Autodesk Inventor part; units mm, degrees
ref_plane "YZ Plane" through (0, 0, 0) normal (1, 0, 0) x (0, 1, 0)
ref_plane "XZ Plane" through (0, 0, 0) normal (0, 1, 0) x (-1, 0, 0)
ref_plane "XY Plane" through (0, 0, 0) normal (0, 0, 1) x (1, 0, 0)
sketch "Sketch1" plane through (0, 0, 0) normal (0, 0, 1) x (1, 0, 0)
  arc A0 (0, 10) -> (100, 10) centre (50, 130) ccw
  line L0 (0, 55) -> (13, 55)
  line L1 (13, 55) -> (13, 25)
  line L2 (13, 25) -> (0, 25)
  line L3 (13, 47.5) -> (39, 47.5)
  line L4 (39, 47.5) -> (39, 46)
  line L5 (39, 46) -> (13, 46)
  line L6 (13, 46) -> (13, 47.5)
  line L7 (13, 34) -> (39, 34)
  line L8 (39, 34) -> (39, 32.5)
  line L9 (39, 32.5) -> (13, 32.5)
  line L10 (13, 46) -> (14, 46)
  line L11 (14, 46) -> (14, 44)
  line L12 (14, 44) -> (13, 44)
  line L13 (13, 44) -> (13, 46)
  line L14 (13, 34) -> (14, 34)
  line L15 (14, 34) -> (14, 36)
  line L16 (14, 36) -> (13, 36)
  line L17 (13, 36) -> (13, 34)
  line L18 (30, 150) -> (32, 142)
  arc A1 (32, 142) -> (50, 141) centre (50, 303.5) ccw
  line L19 (100, 55) -> (87, 55)
  line L20 (87, 55) -> (87, 25)
  line L21 (87, 25) -> (100, 25)
  line L22 (87, 47.5) -> (61, 47.5)
  line L23 (61, 47.5) -> (61, 46)
  line L24 (61, 46) -> (87, 46)
  line L25 (87, 46) -> (87, 47.5)
  line L26 (61, 34) -> (61, 32.5)
  line L27 (87, 34) -> (61, 34)
  line L28 (61, 32.5) -> (87, 32.5)
  line L29 (87, 46) -> (86, 46)
  line L30 (86, 46) -> (86, 44)
  line L31 (86, 44) -> (87, 44)
  line L32 (87, 44) -> (87, 46)
  line L33 (87, 34) -> (86, 34)
  line L34 (86, 34) -> (86, 36)
  line L35 (86, 36) -> (87, 36)
  line L36 (87, 36) -> (87, 34)
  line L37 (70, 150) -> (68, 142)
  arc A2 (50, 141) -> (68, 142) centre (50, 303.5) ccw
  arc A3 (100, 55) -> (80, 150) centre (-148.869, 52.2118) ccw
  line L38 (70, 150) -> (80, 150)
  line L39 (20, 150) -> (30, 150)
  line L40 (100, 25) -> (100, 10)
  line L41 (0, 10) -> (0, 25)
  circle A4 centre (25.0045, 134) radius 1.5 construction
  circle A5 centre (74.7045, 134) radius 1.5 construction
  line L42 (16.9872, 134) -> (99.6032, 134) construction
  line L43 (12.0158, 134) -> (23.5045, 134)
  line L44 (74.7045, 134) -> (86.1932, 134)
  circle A6 centre (25.0045, 134) radius 2
  circle A7 centre (74.7045, 134) radius 2
  circle A8 centre (14.98, 88.58) radius 1.5 construction
  circle A9 centre (86.52, 88.58) radius 1.5 construction
  line L45 (16.652, 88.58) -> (99.2681, 88.58) construction
  line L46 (2.6559, 88.58) -> (13.48, 88.58)
  line L47 (86.52, 88.58) -> (97.3441, 88.58)
  circle A10 centre (14.98, 88.58) radius 2
  circle A11 centre (86.52, 88.58) radius 2
  line L48 (13, 50.0336) -> (87, 50.0336) construction
  line L49 (50, 50.0336) -> (50, 74.1687) construction
  arc A12 (20, 150) -> (0, 55) centre (248.869, 52.2118) ccw
  line L50 (0, 27.09) -> (23.905, 27.09)
  circle A13 centre (25.405, 27.09) radius 1.5 construction
  circle A14 centre (25.405, 27.09) radius 2
  circle A15 centre (76.095, 27.09) radius 1.5 construction
  circle A16 centre (76.095, 27.09) radius 2
  line L51 (30.9298, 27.09) -> (113.5459, 27.09) construction
  line L52 (76.095, 27.09) -> (100, 27.09)
  point P0 (0, 0)
  point P1 (75, 150)
  point P2 (50.8983, 94.4188)
  point P3 (62.5692, 16.9025)
  dimension "d68" = 3
  dimension "d74" = 3
  dimension "d80" = 3
  dimension "d10" = 10
  dimension "d12" = 30
  dimension "d13" = 13
  dimension "d14" = 15
  dimension "d15" = 26
  dimension "d16" = 1.5
  dimension "d19" = 26
  dimension "d20" = 1.5
  dimension "d23" = 7.5
  dimension "d24" = 12
  dimension "d25" = 1
  dimension "d26" = 2
  dimension "d27" = 1
  dimension "d28" = 2
  dimension "d35" = 10
  dimension "d69" = 3
  dimension "d70" = 46.7
  dimension "d71" = 16
  dimension "d72" = 4
  dimension "d73" = 4
  dimension "d75" = 3
  dimension "d76" = 68.54
  dimension "d77" = 4
  dimension "d78" = 4
  dimension "d79" = 45.42
  dimension "d81" = 3
  dimension "d83" = 4
  dimension "d84" = 4
  dimension "d86" = 61.49
  dimension "d107" = 46.69
extrude "Extrusion1" add sketch "Sketch1" along normal blind 10 contours L1 L7 L8 L9 | L28 L26 L27 L20 | L1 L16 L15 L7 | L27 L34 L35 L20 | L1 L5 L11 L12 | L31 L30 L24 L20 | L1 L3 L4 L5 | L24 L23 L22 L20
extrude "Extrusion3" add sketch "Sketch1" along normal blind 3 contours L41 L2 L1 L9 L8 L7 L15 L16 L12 L11 L5 L4 L3 L0 A12 L39 L18 A1 A2 L37 L38 A3 L19 L20 L22 L23 L24 L30 L31 L35 L34 L27 L26 L28 L21 L40 A0
sketch "Sketch2" plane through (0, 0, 3) normal (0, 0, 1) x (1, 0, 0)
  line L0 (39, 34) -> (14, 34)
  line L1 (17.3, 34) -> (16.3, 34)
  line L2 (16.3, 34) -> (16.3, 36)
  line L3 (16.3, 36) -> (17.3, 36)
  line L4 (17.3, 36) -> (17.3, 34)
  line L5 (14, 34) -> (14, 36)
  line L6 (61, 46) -> (86, 46)
  line L7 (83.7, 46) -> (82.7, 46)
  line L8 (82.7, 46) -> (82.7, 44)
  line L9 (82.7, 44) -> (83.7, 44)
  line L10 (83.7, 44) -> (83.7, 46)
  line L11 (86, 46) -> (86, 44)
  point P0 (0, 0)
  point P1 (14, 35)
  dimension "d89" = 1
  dimension "d90" = 2
  dimension "d91" = 2.3
  dimension "d92" = 1
  dimension "d93" = 2
  dimension "d94" = 2.3
extrude "Extrusion4" add sketch "Sketch2" along normal blind 1.5
extrude "Extrusion5" add sketch "Sketch1" along normal blind 24 contours A16 | A11 | A7 | A6 | A10 | A14
sketch "Sketch4" plane through (74.7045, 134, 24) normal (0, 0, 1) x (1, 0, 0)
  circle A0 centre (-49.7, 0) radius 2
  circle A1 centre (-49.7, 0) radius 1.5
  circle A2 centre (0, 0) radius 2
  circle A3 centre (0, 0) radius 1.5
  circle A4 centre (-59.7245, -45.42) radius 2
  circle A5 centre (-59.7245, -45.42) radius 1.5
  circle A6 centre (11.8155, -45.42) radius 2
  circle A7 centre (11.8155, -45.42) radius 1.5
  circle A8 centre (1.3905, -106.91) radius 2
  circle A9 centre (1.3905, -106.91) radius 1.5
  circle A10 centre (-49.2995, -106.91) radius 2
  circle A11 centre (-49.2995, -106.91) radius 1.5
  point P0 (-74.7045, -134)
  dimension "d99" = 3
  dimension "d100" = 3
  dimension "d101" = 3
  dimension "d102" = 3
  dimension "d103" = 3
  dimension "d104" = 3
extrude "Extrusion6" add sketch "Sketch4" along normal blind 2 contours A1 | A3 | A5 | A7 | A9 | A11
sketch "Sketch5" plane through (0, 0, 3) normal (0, 0, 1) x (1, 0, 0)
  circle A0 centre (50, 124.26) radius 7
  point P0 (0, 0)
  dimension "d108" = 14
extrude "Extrusion7" cut sketch "Sketch5" against normal blind 10
Geometry check sheet. Reference: the model listing, model coordinates, mm. A direction names the side the tool comes from. Round coordinates to 2 decimals unless told otherwise and drop trailing zeros. Loops run counter-clockwise (first coordinate to the right, second up) from the corner with the lowest first, then second, coordinate; pieces in that order, holes last. Notation, with made-up numbers: (18, -40) - (38, -40) arc R32 cw to (38, -5) - close; hole circle Ø6 at (20, 61.25). An arc over 180 degrees is marked (long way). One line per question, with ' | ' between items. Start each with the question number.
1. Cross-section at B-B on y = 124.26. Record the cut outline in (x, z), then the cut area to 3 significant figures.
2. Scan lines: line 1 (Y direction, x = 50, z = 2.2); line 2 (Y direction, x = 29, z = 3.75); line 3 (Z direction, x = 46.5, y = 17.5). Record each from-to range of solid material in increasing order. Write a range as [from, to].
3. Cross-section at D-D on y = 88.58. Record the cut outline in (x, z), then the cut area to 3 significant figures.
4. Draft check along Y on faces 4 (the face through (25, 150, 1)), 5 (the face through (6, 55, 1)), 6 (the face through (24, 28, 24)), 7 (the face through (86, 89, 26)). Enter one of: released by +Y, released by -Y, zero draft, split by the parting line, or undercut.
5. Tool access check on faces 1 (the face through (75, 134, 26)), 2 (the face through (26, 47.5, 6)), 3 (the face through (74, 34, 6)). Record the directions out of +Z, -Z, +X, -X, +Y, -Y that give a thin tool (end or side, any length) a straight path to the whole face; none if there is none.
6. Cross-section at A-A on z = 18.75. Record the cut outline in (x, y) (1 decimal), then the cut area to 3 significant figures.
7. Depth check by flat-ended pin: pin 1 (3.5 mm diameter, centred on x = 32, z = 6.5, fed in from -Y); pin 2 (1.2 mm diameter, centred on y = 35, z = 3.5, fed in from -X); pin 3 (1.8 mm diameter, centred on x = 30, y = 34.5, fed in from +Z). Enter the tip coordinate at first touch or a pass-through.
8. Cross-section at C-C on x = 52. Record the cut outline in (y, z), then the cut area to 3 significant figures.
Taken from the geometry:
1) outline: (10.64, 0) - (43, 0) - (43, 3) - (10.64, 3) - close; (57, 0) - (89.36, 0) - (89.36, 3) - (57, 3) - close | area: 194 mm²
2) line 1: [0, 117.26], [131.26, 141] | line 2: [32.5, 34], [46, 47.5] | line 3: [0, 3]
3) outline: (2.66, 0) - (97.34, 0) - (97.34, 3) - (88.52, 3) - (88.52, 24) - (88.02, 24) - (88.02, 26) - (85.02, 26) - (85.02, 24) - (84.52, 24) - (84.52, 3) - (16.98, 3) - (16.98, 24) - (16.48, 24) - (16.48, 26) - (13.48, 26) - (13.48, 24) - (12.98, 24) - (12.98, 3) - (2.66, 3) - close | area: 464 mm²
4) face 4: released by +Y | face 5: undercut | face 6: undercut | face 7: zero draft
5) face 1: +Z, +X, -X, +Y, -Y | face 2: +Z, +X, -X | face 3: +Z
6) outline: circle Ø4 at (15, 88.6); circle Ø4 at (25, 134); circle Ø4 at (25.4, 27.1); circle Ø4 at (74.7, 134); circle Ø4 at (76.1, 27.1); circle Ø4 at (86.5, 88.6) | area: 75.4 mm²
7) pin 1: y = 32.5 | pin 2: x = 13 | pin 3: z = 10
8) outline: (0.02, 0) - (117.55, 0) - (117.55, 3) - (0.02, 3) - close; (130.97, 0) - (141.01, 0) - (141.01, 3) - (130.97, 3) - close | area: 383 mm²
